Solid Edge part; units mm, degrees
sketch "Sketch1" plane through (0, 0, 0) normal (0, 0, 1) x (1, 0, 0)
  line L0 (-12.5, 28) -> (-12.5, -28)
  line L1 (-12.5, -28) -> (12.5, -28)
  line L2 (12.5, -28) -> (12.5, 28)
  line L3 (12.5, 28) -> (-12.5, 28)
extrude "Protrusion1" add sketch "Sketch1" along normal blind 7
sketch "Sketch2" plane through (0, 0, 0) normal (0, 0, 1) x (1, 0, 0)
  line L0 (-12.5, -28) -> (12.5, -28) construction
  line L1 (5.5, -37.5) -> (5.5, 37.5)
  line L2 (-5.5, -37.5) -> (5.5, -37.5)
  line L3 (-5.5, 37.5) -> (-5.5, -37.5)
  line L4 (-1.5, -33.5) -> (-1.5, -30.5)
  line L5 (1.5, -30.5) -> (1.5, -33.5)
  arc A0 (-1.5, -30.5) -> (1.5, -30.5) centre (0, -30.5) cw
  arc A1 (1.5, -33.5) -> (-1.5, -33.5) centre (0, -33.5) cw
  line L6 (-1.5, 30.5) -> (-1.5, 33.5)
  line L7 (1.5, 33.5) -> (1.5, 30.5)
  arc A2 (1.5, 30.5) -> (-1.5, 30.5) centre (0, 30.5) cw
  arc A3 (-1.5, 33.5) -> (1.5, 33.5) centre (0, 33.5) cw
  line L8 (12.5, 28) -> (-12.5, 28) construction
  line L9 (-5.5, 37.5) -> (-5.5, -37.5) construction
  line L10 (5.5, 37.5) -> (-5.5, 37.5)
  line L11 (5.5, -37.5) -> (5.5, 37.5) construction
extrude "ExtrudedProtrusion_2" add sketch "Sketch2" along normal blind 3.5
properties material "Polycarbonate"
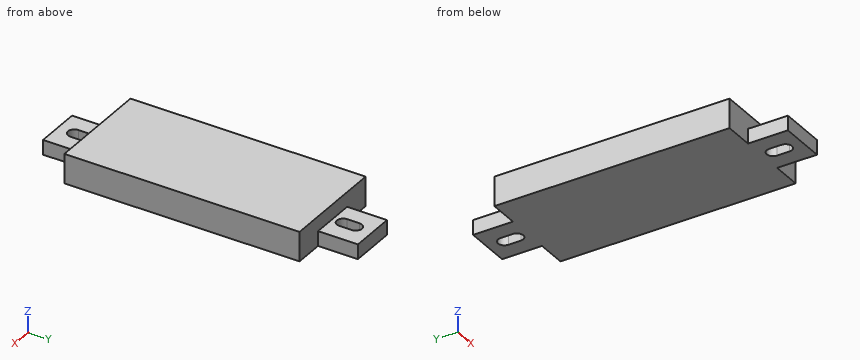
Here's how the part is built. I have some questions about the finished solid (model axes, mm). Coordinates: 2 decimals unless noted, no trailing zeros. Order: outer loops, then holes, each group sorted by start corner. A loop starts at its lowest first (then second) coordinate and runs counter-clockwise, first axis right, second up. Notation, with made-up numbers: M -9,74.25 L 42,74.25 A10 ccw 42,81.25 Z; hole C 29.5,-6 d4. An arc over 180 degrees is marked long. Answer as a JSON object with one key per item and string values. Group by question number.
(1) Suppose I cut it at C-C, the plane z = 4.25. Please give me the cut outline in (x, y).
(2) For pin 1 (1 mm diameter, centred on y = 31, z = 2, fed in from +X); pin 2 (7.5 mm diameter, centred on x = -1.5, y = -31.5, fed in from +Z); pin 3 (4 mm diameter, centred on y = -31.5, z = 2, fed in from -X); pin 4 (3 mm diameter, centred on x = 1, y = 31.5, fed in from +Z), each with a flat end and sliding along its axis, tell me the tip position at first contact or that it passes through.
(3) Suppose I cut it at B-B, the plane x = 3.5. Please give me the cut outline in (y, z).
(4) I need wall thicknesses on probe 1 along X at (y, z) = (-32, 1.5); probe 2 along Y at (x, z) = (11.25, 6); probe 3 along Z at (x, y) = (0.75, 29). Which ranges of each line are inside material? Lowest first, please.
(5) Suppose I cut it at D-D, the plane x = 6.5. Please give me the cut outline in (y, z), then the cut area to 3 significant figures.
(6) Suppose I cut it at A-A, the plane x = 0. Please give me the cut outline in (y, z).
Values found:
{
 "1": {"outline": "M -12.5,-28 L 12.5,-28 L 12.5,28 L -12.5,28 Z"},
 "2": {"pin 1": "stops at x = 5.5", "pin 2": "stops at z = 7", "pin 3": "stops at x = -5.5", "pin 4": "stops at z = 3.5"},
 "3": {"outline": "M -37.5,0 L 37.5,0 L 37.5,3.5 L 28,3.5 L 28,7 L -28,7 L -28,3.5 L -37.5,3.5 Z"},
 "4": {"probe 1": "x = -5.5 to -1.5, 1.5 to 5.5", "probe 2": "y = -28 to 28", "probe 3": "z = 0 to 3.5"},
 "5": {"outline": "M -28,0 L 28,0 L 28,7 L -28,7 Z", "area": "392 mm^2"},
 "6": {"outline": "M -37.5,0 L -35,0 L -35,3.5 L -37.5,3.5 Z; M -29,0 L 29,0 L 29,3.5 L 28,3.5 L 28,7 L -28,7 L -28,3.5 L -29,3.5 Z; M 35,0 L 37.5,0 L 37.5,3.5 L 35,3.5 Z"}
}
